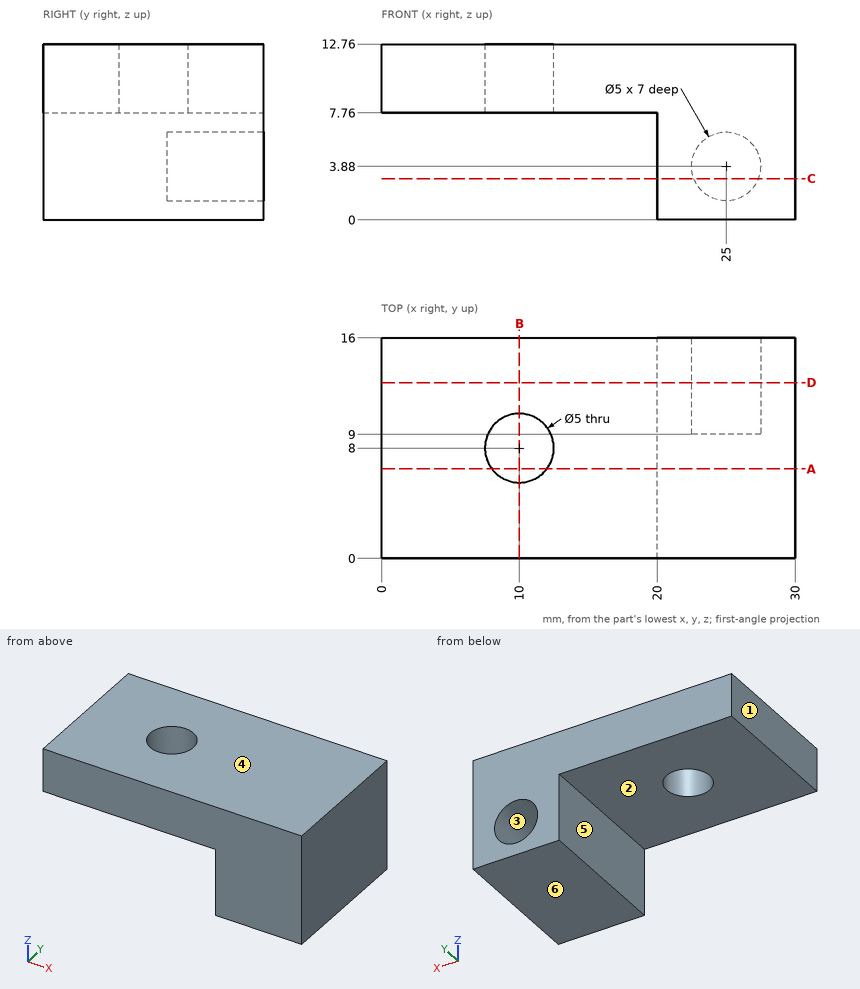
Design review of the part shown in the three views and the two pictorial views. Dimensions are in mm from the part's minimum x, y and z. A direction names the side the tool comes from. Round coordinates to 2 decimals unless told otherwise and drop trailing zeros. Write each loop counter-clockwise with the first axis right and the second up, starting at its lowest first coordinate (ties: lowest second). Pieces come first, ordered by that corner, then holes. Notation, with made-up numbers: M 4.25,-35.5 L 9.25,-35.5 A20 cw 9.25,-28.5 Z; hole C -24.5,53.25 d8. An arc over 180 degrees is marked long. Use a Markdown table: item, result. Add a question column.
Q1. We need section B-B, the plane x = 10. State the section outline as (y, z) points.
Q2. To check wall thickness, follow line 1 (X direction, y = 14.25, z = 3.88); line 2 (Y direction, x = 10, z = 11.5); line 3 (Z direction, x = 25, y = 10.5). State the ranges of each line that lie inside material, in increasing order.
Q3. Machinability: for the marked faces 5 and 6, which of the approach directions +Z, -Z, +X, -X, +Y, -Y give a long, thin tool a straight path to every point of the face, cutting with its end or side? Answer none if there is none.
Q4. Insertion check: pin 1 (2 mm diameter, centred on x = 5.5, y = 10.5, fed in from -Z); pin 2 (1.5 mm diameter, centred on y = 14, z = 2.5, fed in from -X); pin 3 (6.5 mm diameter, centred on x = 25, z = 3.88, fed in from -Y). Each pin has a flat end and moves straight along its axis. Give the tip position at first contact, or say it passes through.
Q5. The part is to be moulded in two halves that separate along Z. For the marked faces 1, 2, 3 and 4, say which applies: pulls with the +Z half, pulls with the -Z half, needs draft (parallel to the pull), parting line crosses it, or undercut.
Q6. We need section C-C, the plane z = 3. State the section outline as (x, y) points.
Q7. We need section A-A, the plane y = 6.5. State the section outline as (x, z) points, plus the area to 3 significant figures.
Q8. We need section D-D, the plane y = 12.75. State the section outline as (x, z) points, plus the area to 3 significant figures.
Findings below:
| question | item | result |
|---|---|---|
| 1 | outline | M 0,7.76 L 5.5,7.76 L 5.5,12.76 L 0,12.76 Z; M 10.5,7.76 L 16,7.76 L 16,12.76 L 10.5,12.76 Z |
| 2 | line 1 | x = 20 to 22.5, 27.5 to 30 |
| 2 | line 2 | y = 0 to 5.5, 10.5 to 16 |
| 2 | line 3 | z = 0 to 1.38, 6.38 to 12.76 |
| 3 | face 5 | -Z, -X, +Y, -Y |
| 3 | face 6 | -Z, +X, -X, +Y, -Y |
| 4 | pin 1 | stops at z = 7.76 |
| 4 | pin 2 | stops at x = 20 |
| 4 | pin 3 | stops at y = 0 |
| 5 | face 1 | needs draft |
| 5 | face 2 | pulls with the -Z half |
| 5 | face 3 | undercut |
| 5 | face 4 | pulls with the +Z half |
| 6 | outline | M 20,0 L 30,0 L 30,16 L 27.34,16 L 27.34,9 L 22.66,9 L 22.66,16 L 20,16 Z |
| 7 | outline | M 0,7.76 L 8,7.76 L 8,12.76 L 0,12.76 Z; M 12,7.76 L 20,7.76 L 20,0 L 30,0 L 30,12.76 L 12,12.76 Z |
| 7 | area | 208 mm² |
| 8 | outline | M 0,7.76 L 20,7.76 L 20,0 L 30,0 L 30,12.76 L 0,12.76 Z; hole C 25,3.88 d5 |
| 8 | area | 208 mm² |
